Design review of the part built by this model. Coordinates are the model's own, in mm. Face numbers are marked on the shaded views. Give positions to 0.01 mm unless a question says otherwise; leave off trailing zeros. Write each loop counter-clockwise with the first axis right and the second up, starting at its lowest first coordinate (ties: lowest second). Pieces come first, ordered by that corner, then holes.
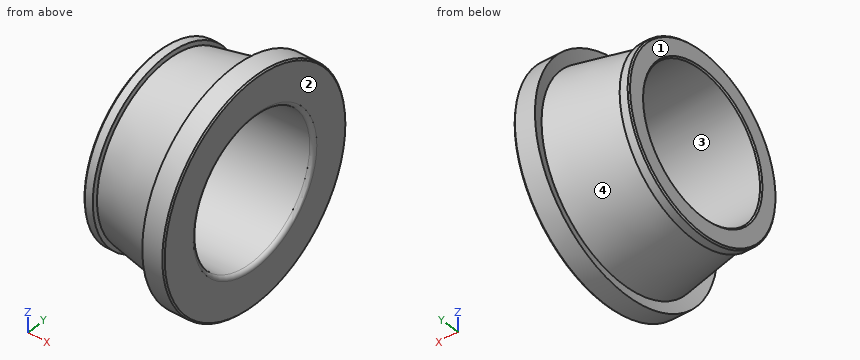
Solid Edge part; units mm, degrees
sketch "Sketch1" plane through (0, 0, 0) normal (0, 0, 1) x (1, 0, 0)
  line L0 (0, 11.2) -> (0.2, 11)
  line L1 (0.2, 11) -> (14.4, 11)
  arc A0 (14.4, 11) -> (15, 11.6) centre (14.4, 11.6) ccw
  line L2 (15, 11.6) -> (15, 16.95)
  line L3 (15, 16.95) -> (14.8, 17.15)
  line L4 (14.8, 17.15) -> (11.7245, 17.15)
  line L5 (11.7245, 17.15) -> (12.2103, 15.3157)
  line L6 (12.2103, 15.3157) -> (1.585, 13.2504)
  line L7 (1.585, 13.2504) -> (1.4275, 13.845)
  line L8 (1.4275, 13.845) -> (0.2, 13.845)
  line L9 (0.2, 13.845) -> (0, 13.645)
  line L10 (0, 13.645) -> (0, 11.2)
revolve "RevolvedProtrusion1" add sketch "Sketch1" angle 360 about axis through (15, 0, 0) along (-1, 0, 0)
properties part number "320/22 X_ir"
(1) Consider section D-D, the plane x = 10.75. Give the boundary of the cut face in (y, z).
Resolved:
outline: circle Ø30.06 at (0, 0); hole circle Ø22 at (0, 0)
(2) Consider section C-C, the plane x = 6.5. Give the boundary of the cut face in (y, z), then the cut area to 3 significant figures.
Resolved:
outline: circle Ø28.41 at (0, 0); hole circle Ø22 at (0, 0)
area: 254 mm2
(3) To check wall thickness, follow L1, parallel to Z at x = 11, y = 8; L2, parallel to Y at x = 7, z = 2; L3, parallel to Z at x = 3.75, y = -7. State the ranges of each line that lie inside material, in increasing order.
Resolved:
L1: z = -12.78 to -7.55, 7.55 to 12.78
L2: y = -14.16 to -10.82, 10.82 to 14.16
L3: z = -11.74 to -8.49, 8.49 to 11.74
(4) Clearance check with flat-ended pins moving along their axes: P1, Ø1.5, axis at x = 8, z = 5.5, coming from the -Y side; P2, Ø4, axis at y = 8.5, z = 4.5, coming from the -X side; P3, Ø6, axis at x = 2, y = -4.5, coming from the +Z side; P4, Ø3, axis at x = 2, y = -6, coming from the -Z side. State where each tip first meets the part, or that it passes through.
Resolved:
P1: stops at y = -13.74
P2: stops at x = 0
P3: stops at z = 13.76
P4: stops at z = -13.05
(5) Mouldability with a two-part tool opening along X and no side actions: class the marked faces 1, 2, 3 and 4 as pulls with the +X half, pulls with the -X half, needs draft (parallel to the pull), parting line crosses it, or undercut.
Resolved:
face 1: pulls with the -X half
face 2: pulls with the +X half
face 3: needs draft
face 4: undercut
